The listing builds one solid part. Answer for the finished solid, in the listing's coordinates (mm). A direction names the side the tool comes from. Round coordinates to 2 decimals unless told otherwise and drop trailing zeros. Return JSON: item names as keys, results as strings. Group by question number.
(1) Consider line 1 (Y direction, x = 8, z = 0); line 2 (X direction, y = -29.5, z = 63); line 3 (X direction, y = 18, z = 11). Determine where each line is inside the solid, lowest interval first. Write a range as [from, to].
(2) Each of these flat-tipped pins is pushed along its axis until it touches: pin 1 (5 mm diameter, centred on x = 72.5, z = 78.5, fed in from +Y); pin 2 (6 mm diameter, centred on y = -25.5, z = 63, fed in from +X); pin 3 (1.5 mm diameter, centred on x = 38.5, z = 0, fed in from -Y). Where does it stop, or does it pass through?
(3) Determine the mould class of faces 1 (the face through (52, -97, -12.57)), 2 (the face through (43.87, -98.94, 38.94)), 3 (the face through (148.27, 115.87, 0.79)) for opening direction X: +X half, -X half, draft (parallel to the pull), parting line (faces both ways), or undercut.
(4) Which of the six approach directions +Z, -Z, +X, -X, +Y, -Y give full straight-line access (tool end or side, diameter ignored) to faces 4 (the face through (-103.862, 39.604, -11.959)), 5 (the face through (-82.64, 32.92, 75.53)), 6 (the face through (98, -68, 89.03))?
from build123d import *

# Parameters (mm, degrees)
F2_R    = 5
F3_SIZE = 2


with BuildPart() as f1:
    # F0 (on Front) → F1 (revolve)
    with BuildSketch(Plane.XZ):
        Polygon((-79.4498865843, -12.5698290182), (-79.4498865843, 89.0301709818), (-81.0498865843, 89.0301709818), (-87.6998865843, 83.9274465117), (-87.6998865843, 67.3713907599), (-101.1498865843, 15.8301709818), (-149.5498865843, 15.8301709818), (-149.5498865843, -10.9698290182), (-109.9510937929, -10.9698290182), (-109.9498865843, -12.5698290182), align=None)
    revolve(axis=Axis((21.9001134157, 0, 0.9622275829), (0, 0, -1)))

    # F2
    f2_edges = [f1.edges().sort_by_distance(p)[0] for p in [
        (193.350113, 0, 15.830171),
    ]]
    fillet(f2_edges, radius=F2_R)

    # F3
    f3_edges = [f1.edges().sort_by_distance(p)[0] for p in [
        (193.350113, 0, -10.969829),
    ]]
    chamfer(f3_edges, length=F3_SIZE)


solid = f1.part
Answer below:
{
 "1": {"line 1": "y = [-170.89, -100.39], [100.39, 170.89]", "line 2": "x = [-84.84, -75.06], [118.86, 128.64]", "line 3": "x = [-148.6, -77.84], [121.64, 192.4]"},
 "2": {"pin 1": "stops at y = 98.48", "pin 2": "stops at x = 130.72", "pin 3": "stops at y = -170.72"},
 "3": {"face 1": "draft", "face 2": "undercut", "face 3": "parting line"},
 "4": {"face 4": "-Z", "face 5": "+Z", "face 6": "+Z, +X, -X, +Y, -Y"}
}
